from build123d import *

# Parameters (mm, degrees)
SURFACE_EXTRUDE2_1_DEPTH = 6
THICKEN2_T1              = 1


with BuildPart() as body_1:
    # Surface-Extrude2: a surface, the sketch's curves swept straight by 6 mm
    with BuildLine(Plane.XY, mode=Mode.PRIVATE) as surface_extrude2_1_path:
        Line((-69, 0.25), (-12, 0.25))
        ThreePointArc((-12, 0.25), (-6.652714965, 8.114011059), (-15.931902505, 10.195550345))
        Line((-15.931902505, 10.195550345), (-19.243429867, 7.092118933))
        ThreePointArc((-19.243429867, 7.092118933), (-21.5, 6.2), (-23.756570133, 7.092118933))
        Line((-23.756570133, 7.092118933), (-27.068097495, 10.195550345))
        ThreePointArc((-27.068097495, 10.195550345), (-31.500549593, 11.72817162), (-35.6, 9.45))
        Line((-35.6, 9.45), (-37.34, 7.13))
        ThreePointArc((-37.34, 7.13), (-40.5, 5.55), (-43.66, 7.13))
        Line((-43.66, 7.13), (-45.4, 9.45))
        ThreePointArc((-45.4, 9.45), (-49.499450407, 11.72817162), (-53.931902505, 10.195550345))
        Line((-53.931902505, 10.195550345), (-57.243429867, 7.092118933))
        ThreePointArc((-57.243429867, 7.092118933), (-59.5, 6.2), (-61.756570133, 7.092118933))
        Line((-61.756570133, 7.092118933), (-65.068097495, 10.195550345))
        ThreePointArc((-65.068097495, 10.195550345), (-74.347285035, 8.114011059), (-69, 0.25))
    surface_extrude2_1 = Shell.extrude(surface_extrude2_1_path.wire(), (0 * SURFACE_EXTRUDE2_1_DEPTH, 0 * SURFACE_EXTRUDE2_1_DEPTH, 1 * SURFACE_EXTRUDE2_1_DEPTH))
    add(Solid.thicken(surface_extrude2_1, THICKEN2_T1))


solid = body_1.part
Verification items for the finished model (mm, model axes). A direction names the side the tool comes from. Coordinates: 2 decimals unless noted, no trailing zeros. Write each loop counter-clockwise with the first axis right and the second up, starting at its lowest first coordinate (ties: lowest second). Pieces come first, ordered by that corner, then holes. Notation, with made-up numbers: M 55.25,35 L 78.25,35 A20 ccw 78.25,55 Z; hole C 40.25,19.25 d7. An arc over 180 degrees is marked long. One line per question, with ' | ' between items.
1) Depth check by flat-ended pin: pin 1 Ø5.5 at (x, y) = (-69, 6) entering from -Z; pin 2 Ø2 at (y, z) = (3.5, 2) entering from +X; pin 3 Ø1.8 at (x, z) = (-44, 2.5) entering from +Y. Enter the tip coordinate at first touch or a pass-through.
Solutions:
pin 1: through | pin 2: x = -6.45 | pin 3: y = 8.78
2) Sectioned sample at B-B on z = 4.4. Record the cut outline in (x, y), then the cut area to 3 significant figures.
Solutions:
outline: M -69,0.25 L -12,0.25 A5.75 ccw long -15.93,10.2 L -19.24,7.09 A3.3 cw -23.76,7.09 L -27.07,10.2 A5.75 ccw -35.6,9.45 L -37.34,7.13 A3.95 cw -43.66,7.13 L -45.4,9.45 A5.75 ccw -53.93,10.2 L -57.24,7.09 A3.3 cw -61.76,7.09 L -65.07,10.2 A5.75 ccw long Z; hole M -69,1.25 L -12,1.25 A4.75 ccw long -15.25,9.47 L -18.56,6.36 A4.3 cw -24.44,6.36 L -27.75,9.47 A4.75 ccw -34.8,8.85 L -36.54,6.53 A4.95 cw -44.46,6.53 L -46.2,8.85 A4.75 ccw -53.25,9.47 L -56.56,6.36 A4.3 cw -62.44,6.36 L -65.75,9.47 A4.75 ccw long Z | area: 159 mm^2
3) Access from +Z, -Z, +X, -X, +Y, -Y to the whole of each face (thin tool, end or side, straight path). Record for faces 1 (the face through (-63.389, 8.622, 2.958)), 2 (the face through (-41, 5, 6)), 3 (the face through (-45.318, 7.674, 2.958)).
Solutions:
face 1: +Z, -Z, +Y | face 2: +Z, +X, -X, +Y, -Y | face 3: +Z, -Z
4) Sectioned sample at C-C on y = 3.25. Record the cut outline in (x, z).
Solutions:
outline: M -74.05,0 L -72.87,0 L -72.87,6 L -74.05,6 Z; M -8.13,0 L -6.95,0 L -6.95,6 L -8.13,6 Z
5) Sectioned sample at A-A on x = -59.5. Record the cut outline in (y, z).
Solutions:
outline: M 0.25,0 L 1.25,0 L 1.25,6 L 0.25,6 Z; M 5.2,0 L 6.2,0 L 6.2,6 L 5.2,6 Z
6) Material ranges on L1, parallel to Y at x = -69, z = 3.6; L2, parallel to X at y = 6, z = 4.3, recorded low to high.
Solutions:
L1: 0.25 to 1.25, 10.75 to 11.75 | L2: -74.75 to -73.75, -62 to -57, -44 to -42.33, -38.67 to -37, -24 to -19, -7.25 to -6.25
7) Release check for a two-part mould opening along Y. For faces 4 (the face through (-54.881, 7.936, 2.958)), 5 (the face through (-55.56, 8.67, 2.96)), 6 (the face through (-16.881, 7.936, 2.958)), 7 (the face through (-41, 5, 0)) record: +Y half, -Y half, draft (parallel to the pull), parting line (faces both ways), or undercut.
Solutions:
face 4: undercut | face 5: +Y half | face 6: undercut | face 7: draft
